Design review of the part built by this model. Coordinates are the model's own, in mm. A direction names the side the tool comes from. Give positions to 0.01 mm unless a question says otherwise; leave off trailing zeros. Order: outer loops, then holes, each group sorted by start corner. A loop starts at its lowest first (then second) coordinate and runs counter-clockwise, first axis right, second up. Notation, with made-up numbers: (65, 19.25) -> (94, 19.25) arc R35 ccw to (94, 57.25) -> close; hole circle Ø3 at (71, 30.25). An arc over 180 degrees is marked (long way). One line per item, written item: value.
from build123d import *

# Parameters (mm, degrees)
F0_R     = 5
F1_DEPTH = 20
F2_R     = 7.5
F2_R_2   = 4.5
F3_DEPTH = 12
F4_DEPTH = 25
F5_SIZE2 = 1
F5_SIZE  = 1


with BuildPart() as f1:
    # F0 (on Front) → F1 (new body)
    with BuildSketch(Plane.XZ):
        Polygon((0, 45), (60, 0), (255, 0), (255, 160), (0, 160), align=None)
        with Locations((127.5, 15)):
            Circle(F0_R, mode=Mode.SUBTRACT)
        with BuildLine():
            ThreePointArc((35, 32.5), (17.5, 50), (35, 67.5))
            Line((35, 67.5), (182.5, 67.5))
            ThreePointArc((182.5, 67.5), (193.106602, 71.893398), (197.5, 82.5))
            Line((197.5, 82.5), (197.5, 112.5))
            ThreePointArc((197.5, 112.5), (215, 130), (232.5, 112.5))
            Line((232.5, 112.5), (232.5, 82.5))
            ThreePointArc((232.5, 82.5), (217.855339, 47.144661), (182.5, 32.5))
            Line((182.5, 32.5), (35, 32.5))
        make_face(mode=Mode.SUBTRACT)
        with Locations((127.5, 145)):
            Circle(F0_R, mode=Mode.SUBTRACT)
    extrude(amount=-F1_DEPTH)

    # F2 (on face) → F3 (cut)
    with BuildSketch(Plane.XZ):
        with Locations((20, 145)):
            Circle(F2_R)
        with Locations((20, 145)):
            Circle(F2_R_2, mode=Mode.SUBTRACT)
        with Locations((235, 145)):
            Circle(F2_R)
        with Locations((235, 145)):
            Circle(F2_R_2, mode=Mode.SUBTRACT)
        with Locations((235, 15)):
            Circle(F2_R)
        with Locations((235, 15)):
            Circle(F2_R_2, mode=Mode.SUBTRACT)
        with Locations((87.5, 15)):
            Circle(F2_R)
        with Locations((87.5, 15)):
            Circle(F2_R_2, mode=Mode.SUBTRACT)
    extrude(amount=-F3_DEPTH, mode=Mode.SUBTRACT)

    # F2 (on face) → F4 (cut)
    with BuildSketch(Plane.XZ):
        with Locations((20, 145)):
            Circle(F2_R_2)
        with Locations((235, 145)):
            Circle(F2_R_2)
        with Locations((87.5, 15)):
            Circle(F2_R_2)
        with Locations((235, 15)):
            Circle(F2_R_2)
    extrude(amount=-F4_DEPTH, mode=Mode.SUBTRACT)

    # F5
    f5_edges = [f1.edges().sort_by_distance(p)[0] for p in [
        (157.5, 0, 0),
        (255, 0, 80),
        (127.5, 0, 160),
        (0, 0, 102.5),
        (30, 0, 22.5),
        (108.75, 0, 67.5),
        (17.5, 0, 50),
        (108.75, 0, 32.5),
        (217.855339, 0, 47.144661),
    ]]
    chamfer(f5_edges, length=F5_SIZE, length2=F5_SIZE2)


solid = f1.part
Item 1: Clearance check with flat-ended pins moving along their axes: P1, Ø19.5, axis at x = 87.5, z = 15, coming from the +Y side; P2, Ø5, axis at y = 16, z = 30.5, coming from the -X side; P3, Ø12, axis at x = 235, z = 145, coming from the -Y side; P4, Ø4, axis at y = 13, z = 38.5, coming from the -X side. State where each tip first meets the part, or that it passes through.
Returned:
P1: y = 20
P2: x = 16
P3: y = 12
P4: x = 6
Item 2: Machinability: for faces 3 (the flat face through (232.5, 10, 98)), 4 (the flat face through (255, 10, 79)), 5 (the flat face through (240, 12, 15)), which of the approach directions +Z, -Z, +X, -X, +Y, -Y give a long, thin tool a straight path to every point of the face, cutting with its end or side? Answer none if there is none.
Returned:
face 3: +Y, -Y
face 4: +Z, -Z, +X, +Y, -Y
face 5: -Y
Item 3: Add section C-C on y = 4.25. Give the boundary of the cut face in (x, z), plus the area to 3 significant figures.
Returned:
outline: (0, 45) -> (60, 0) -> (255, 0) -> (255, 160) -> (0, 160) -> close; hole circle Ø15 at (20, 145); hole (35, 32.5) -> (182.5, 32.5) arc R50 ccw to (232.5, 82.5) -> (232.5, 112.5) arc R17.5 ccw to (197.5, 112.5) -> (197.5, 82.5) arc R15 cw to (182.5, 67.5) -> (35, 67.5) arc R17.5 ccw to start; hole circle Ø15 at (87.5, 15); hole circle Ø10 at (127.5, 15); hole circle Ø10 at (127.5, 145); hole circle Ø15 at (235, 15); hole circle Ø15 at (235, 145)
area: 29,600 mm²
Item 4: Draft analysis for pull direction Y (two halves, no side actions). For faces 1 (the cylindrical face through (239.292, 15.944, 16.352)), 2 (the flat face through (126, 0, 99)), state which applies: pulls with the +Y half, pulls with the -Y half, needs draft (parallel to the pull), parting line crosses it, or undercut.
Returned:
face 1: needs draft
face 2: pulls with the -Y half
Item 5: Add section D-D on x = 148. Give the boundary of the cut face in (y, z), plus the area to 3 significant figures.
Returned:
outline: (0, 1) -> (1, 0) -> (20, 0) -> (20, 32.5) -> (1, 32.5) -> (0, 31.5) -> close; (0, 68.5) -> (1, 67.5) -> (20, 67.5) -> (20, 160) -> (1, 160) -> (0, 159) -> close
area: 2,500 mm²
Item 6: Add section B-B on z = 145. Give the boundary of the cut face in (x, y).
Returned:
outline: (0, 1) -> (1, 0) -> (12.5, 0) -> (12.5, 12) -> (15.5, 12) -> (15.5, 20) -> (0, 20) -> close; (24.5, 12) -> (27.5, 12) -> (27.5, 0) -> (122.5, 0) -> (122.5, 20) -> (24.5, 20) -> close; (132.5, 0) -> (227.5, 0) -> (227.5, 12) -> (230.5, 12) -> (230.5, 20) -> (132.5, 20) -> close; (239.5, 12) -> (242.5, 12) -> (242.5, 0) -> (254, 0) -> (255, 1) -> (255, 20) -> (239.5, 20) -> close
Item 7: To check wall thickness, follow line 1 along Z through (x, y) = (235, 17.25); line 2 along Z through (x, y) = (127.5, 11); line 3 along Z through (x, y) = (235, 7.5). State the ranges of each line that lie inside material, in increasing order. Write a range as from..to.
Returned:
line 1: 0..10.5, 19.5..140.5, 149.5..160
line 2: 0..10, 20..32.5, 67.5..140, 150..160
line 3: 0..7.5, 22.5..137.5, 152.5..160
Item 8: Add section A-A on z = 90.5. Give the boundary of the cut face in (x, y).
Returned:
outline: (0, 1) -> (1, 0) -> (196.5, 0) -> (197.5, 1) -> (197.5, 20) -> (0, 20) -> close; (232.5, 1) -> (233.5, 0) -> (254, 0) -> (255, 1) -> (255, 20) -> (232.5, 20) -> close
